```python
from build123d import *

# Parameters (mm, degrees)
SKETCH_1_W          = 25
SKETCH_1_H          = 25
EXTRUDE_1_DEPTH     = 14.5
SKETCH_2_W          = 25
SKETCH_2_H          = 7.25
SKETCH_2_H_2        = 6.5
CUT_EXTRUDE_1_DEPTH = 13
SKETCH_3_W          = 25
SKETCH_3_H          = 0.5
CUT_EXTRUDE_2_DEPTH = 11.6


with BuildPart() as part:
    # Эскиз1 → Бобышка-Вытянуть1 (new body)
    with BuildSketch(Plane.XY):
        with Locations((12.5, 12.5)):
            Rectangle(SKETCH_1_W, SKETCH_1_H)
    extrude(amount=EXTRUDE_1_DEPTH)

    # Эскиз2 → Вырез-Вытянуть1 (cut)
    with BuildSketch(Plane.XY.offset(14.5)):
        with Locations((12.5, 21.375)):
            Rectangle(SKETCH_2_W, SKETCH_2_H)
        with Locations((12.5, 12.5)):
            Rectangle(SKETCH_2_W, SKETCH_2_H_2)
        with Locations((12.5, 3.625)):
            Rectangle(SKETCH_2_W, SKETCH_2_H)
    extrude(amount=-CUT_EXTRUDE_1_DEPTH, mode=Mode.SUBTRACT)

    # Эскиз3 → Вырез-Вытянуть2 (cut)
    with BuildSketch(Plane.XY.offset(1.5)):
        with Locations((12.5, 17.5)):
            Rectangle(SKETCH_3_W, SKETCH_3_H)
        with Locations((12.5, 7.5)):
            Rectangle(SKETCH_3_W, SKETCH_3_H)
    extrude(amount=CUT_EXTRUDE_2_DEPTH, mode=Mode.SUBTRACT)


solid = part.part
```
Check sheet for the modelled part. Datum: model origin and axes. Units: mm. A direction names the side the tool comes from. Give positions to 0.01 mm unless a question says otherwise; leave off trailing zeros. Order: outer loops, then holes, each group sorted by start corner. A loop starts at its lowest first (then second) coordinate and runs counter-clockwise, first axis right, second up. Notation, with made-up numbers: M 73,71.25 L 98,71.25 A22 cw 98,104.25 Z; hole C 35,65 d5. An arc over 180 degrees is marked long. Answer in a Markdown table with one row per item. Add a question column.
Q1. Sectioned sample at B-B, the plane x = 6.5. Record the boundary of the cut face in (y, z).
Q2. Sectioned sample at C-C, the plane y = 14.75. Record the boundary of the cut face in (x, z), and give its area (3 significant figures).
Q3. Sectioned sample at A-A, the plane z = 4. Record the boundary of the cut face in (x, y), and give its area (3 significant figures).
Q4. Thickness scan on L1, parallel to Y at x = 6, z = 9.5; L2, parallel to Z at x = 8.5, y = 2.25. Record the ranges inside material, lowest first.
Q5. Access from +Z, -Z, +X, -X, +Y, -Y to the whole of each face (thin tool, end or side, straight path). Record for faces 1 (the flat face through (12, 17.25, 7)), 2 (the flat face through (12, 9.25, 8)), 3 (the flat face through (12, 17.75, 14)), 4 (the flat face through (12, 7.75, 7)), 5 (the flat face through (12, 7.25, 14)).
Q6. Release check for a two-part mould opening along Y. For faces 6 (the flat face through (12, 15.75, 8)), 7 (the flat face through (12, 0, 1)), 8 (the flat face through (12, 17, 14.5)) record: released by +Y, released by -Y, zero draft, split by the parting line, or undercut.
Q7. Gauge pin test, flat ends, axial feed: pin 1 Ø8.5 at (x, y) = (16, 22.5) entering from +Z; pin 2 Ø3 at (x, z) = (16.5, 7.5) entering from +Y; pin 3 Ø8 at (y, z) = (14.5, 12) entering from -X; pin 4 Ø0.7 at (x, z) = (16.5, 13.5) entering from -Y. Record the tip position at first contact, or that the pin passes through.
Verdict:
| question | item | result |
|---|---|---|
| 1 | outline | M 0,0 L 25,0 L 25,1.5 L 17.25,1.5 L 17.25,13.1 L 17.75,13.1 L 17.75,14.5 L 15.75,14.5 L 15.75,1.5 L 9.25,1.5 L 9.25,14.5 L 7.25,14.5 L 7.25,13.1 L 7.75,13.1 L 7.75,1.5 L 0,1.5 Z |
| 2 | outline | M 0,0 L 25,0 L 25,1.5 L 0,1.5 Z |
| 2 | area | 37.5 mm² |
| 3 | outline | M 0,7.75 L 25,7.75 L 25,9.25 L 0,9.25 Z; M 0,15.75 L 25,15.75 L 25,17.25 L 0,17.25 Z |
| 3 | area | 75.0 mm² |
| 4 | L1 | 7.75 to 9.25, 15.75 to 17.25 |
| 4 | L2 | 0 to 1.5 |
| 5 | face 1 | +X, -X, +Y |
| 5 | face 2 | +Z, +X, -X |
| 5 | face 3 | +Z, +X, -X, +Y |
| 5 | face 4 | +X, -X, -Y |
| 5 | face 5 | +Z, +X, -X, -Y |
| 6 | face 6 | undercut |
| 6 | face 7 | released by -Y |
| 6 | face 8 | zero draft |
| 7 | pin 1 | z = 1.5 |
| 7 | pin 2 | y = 17.25 |
| 7 | pin 3 | x = 0 |
| 7 | pin 4 | y = 7.25 |
